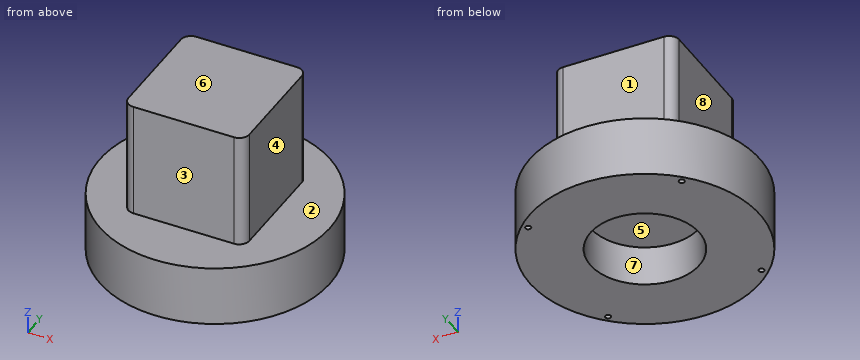
```python
from build123d import *

# Parameters (mm, degrees)
F0_R     = 72.39
F1_DEPTH = 38.1
F2_W     = 76.2
F2_H     = 76.2
F3_DEPTH = 73.025
F4_R     = 6.35
F5_R     = 1.7272
F6_DEPTH = 6.35
F7_R     = 34.29
F8_DEPTH = 25.4


with BuildPart() as f1:
    # F0 (on Top) → F1 (new body)
    with BuildSketch(Plane.XY):
        Circle(F0_R)
    extrude(amount=F1_DEPTH)

    # F2 (on face) → F3 (join)
    with BuildSketch(Plane.XY.offset(38.1)):
        Rectangle(F2_W, F2_H)
    extrude(amount=F3_DEPTH)

    # F4
    f4_edges = [f1.edges().sort_by_distance(p)[0] for p in [
        (-38.1, -38.1, 74.6125),
        (-38.1, 38.1, 74.6125),
        (38.1, -38.1, 74.6125),
        (38.1, 38.1, 74.6125),
    ]]
    fillet(f4_edges, radius=F4_R)

    # F5 (on face) → F6 (cut)
    with BuildSketch(Plane(origin=(0, 0, 0), x_dir=(1, 0, 0), z_dir=(0, 0, -1))):
        with Locations((-48.38113, 48.38113)):
            Circle(F5_R)
        with Locations((-48.38113, -48.38113)):
            Circle(F5_R)
        with Locations((48.38113, -48.38113)):
            Circle(F5_R)
        with Locations((48.38113, 48.38113)):
            Circle(F5_R)
    extrude(amount=-F6_DEPTH, mode=Mode.SUBTRACT)

    # F7 (on face) → F8 (cut)
    with BuildSketch(Plane(origin=(0, 0, 0), x_dir=(1, 0, 0), z_dir=(0, 0, -1))):
        Circle(F7_R)
    extrude(amount=-F8_DEPTH, mode=Mode.SUBTRACT)


solid = f1.part
```
CAD build for the part. Positions are in the model's coordinates, mm. Face numbers are marked on the shaded views. A direction names the side the tool comes from. Coordinates: 2 decimals unless noted, no trailing zeros. Order: outer loops, then holes, each group sorted by start corner. A loop starts at its lowest first (then second) coordinate and runs counter-clockwise, first axis right, second up. Notation, with made-up numbers: M 10.5,-11.75 L 55.5,-11.75 A17 ccw 55.5,-6.75 Z; hole C -31.75,62 d7. An arc over 180 degrees is marked long. Write each question's results on one line, items separated by ' | '. Start each with the question number.
Q1. Flat gauge pins, fed straight in: P1, Ø5, axis at y = -32.5, z = 33.5, coming from the -X side; P2, Ø10, axis at y = 2, z = 54.5, coming from the +X side; P3, Ø4, axis at x = 48.38, y = 48.38, coming from the +Z side. Where does each tip first touch, or does it go through?
Q2. Drill centre lines: probe 1 along Y at (x, z) = (-22, 105); probe 2 along Z at (x, y) = (66, -25.5). Where is each one in solid material? Low to high. Write a range as from..to.
Q3. Cut at A-A (y = 0). List the corners of the cut face in (x, z) (3 decimals), then the cut area to 3 significant figures.
Q4. Cut at D-D (x = -57). List the corners of the cut face in (y, z).
Q5. Cut at C-C (y = -42). List the corners of the cut face in (x, z).
Q6. Pull direction X, two halves, no side cores. Call the marked faces 6, 7 and 8: +X half, -X half, draft (parallel to the pull), parting line (faces both ways), or undercut.
Q7. Which spindle directions (+Z, -Z, +X, -X, +Y, -Y) get a long thin tool onto all of the face, cutting with end or side? Do the marked faces 1, 2, 3, 4 and 5. Say none if no direction does.
Found:
1) P1: x = -65.88 | P2: x = 38.1 | P3: z = 38.1
2) probe 1: -38.1..38.1 | probe 2: 0..38.1
3) outline: M -72.39,0 L -34.29,0 L -34.29,25.4 L 34.29,25.4 L 34.29,0 L 72.39,0 L 72.39,38.1 L 38.1,38.1 L 38.1,111.125 L -38.1,111.125 L -38.1,38.1 L -72.39,38.1 Z | area: 9,340 mm²
4) outline: M -44.62,0 L 44.62,0 L 44.62,38.1 L -44.62,38.1 Z
5) outline: M -58.96,0 L 58.96,0 L 58.96,38.1 L -58.96,38.1 Z
6) face 6: draft | face 7: undercut | face 8: -X half
7) face 1: +Z, +X, -X, +Y | face 2: +Z | face 3: +Z, +X, -X, -Y | face 4: +Z, +X, +Y, -Y | face 5: -Z
